Can you work these out from the model? Positions are in its coordinate system, mm. A direction names the side the tool comes from. Round coordinates to 2 decimals unless told otherwise and drop trailing zeros. Order: outer loops, then holes, each group sorted by start corner. A loop starts at its lowest first (then second) coordinate and runs counter-clockwise, first axis right, second up. Notation, with made-up numbers: M -29.5,43 L -0.5,43 A17 cw -0.5,74 Z; hole C 71.5,-31 d4. An arc over 180 degrees is marked long. One line per question, with ' | ' between items.
```python
from build123d import *

# Parameters (mm, degrees)
SKETCH1_W           = 20
SKETCH1_H           = 20
BOSS_EXTRUDE1_DEPTH = 1
CUT_EXTRUDE1_DEPTH  = 1
FILL_START          = -1
FILL_PATTERN1_DEPTH = 2
SKETCH2_W           = 20
SKETCH2_H           = 20
BOSS_EXTRUDE2_DEPTH = 1


# Read off the part's stored shape, not the designer's step: Fill Pattern1
with BuildPart() as part:
    # Sketch1 → Boss-Extrude1 (new, symmetric)
    with BuildSketch(Plane(origin=(0, 0, 0), x_dir=(1, 0, 0), z_dir=(0, 1, 0))):
        Rectangle(SKETCH1_W, SKETCH1_H)
    extrude(amount=BOSS_EXTRUDE1_DEPTH, both=True)

    # Sketch1<4> → Cut-Extrude1 (cut, symmetric)
    with BuildSketch(Plane(origin=(0, 0, 0), x_dir=(1, 0, 0), z_dir=(0, 1, 0))):
        with BuildLine():
            Line((0.5, 2.5), (0.5, -2.5))
            ThreePointArc((0.5, -2.5), (0, -3), (-0.5, -2.5))
            Line((-0.5, -2.5), (-0.5, 2.5))
            ThreePointArc((-0.5, 2.5), (0, 3), (0.5, 2.5))
        make_face()
    extrude(amount=CUT_EXTRUDE1_DEPTH, both=True, mode=Mode.SUBTRACT)

    # Fill Pattern1 outline → Fill Pattern1 (cut)
    with BuildSketch(Plane(origin=(0, 0, 0), x_dir=(1, 0, 0), z_dir=(0, 1, 0)).offset(FILL_START)):
        with BuildLine():
            Line((0.5, -10), (0.5, -6.160254038))
            ThreePointArc((0.5, -6.160254038), (0, -5.660254038), (-0.5, -6.160254038))
            Line((-0.5, -6.160254038), (-0.5, -10))
            Line((-0.5, -10), (0.5, -10))
        make_face()
        with BuildLine():
            ThreePointArc((2.597603377, -10), (2.5, -9.990381057), (2.402396623, -10))
            Line((2.402396623, -10), (2.597603377, -10))
        make_face()
        with BuildLine():
            Line((-2.597603377, -10), (-2.402396623, -10))
            ThreePointArc((-2.402396623, -10), (-2.5, -9.990381057), (-2.597603377, -10))
        make_face()
        with BuildLine():
            Line((4.5, -6.160254038), (4.5, -10))
            Line((4.5, -10), (5.5, -10))
            Line((5.5, -10), (5.5, -6.160254038))
            ThreePointArc((5.5, -6.160254038), (5, -5.660254038), (4.5, -6.160254038))
        make_face()
        with BuildLine():
            Line((-5.5, -10), (-4.5, -10))
            Line((-4.5, -10), (-4.5, -6.160254038))
            ThreePointArc((-4.5, -6.160254038), (-5, -5.660254038), (-5.5, -6.160254038))
            Line((-5.5, -6.160254038), (-5.5, -10))
        make_face()
        with BuildLine():
            ThreePointArc((7.597603377, -10), (7.5, -9.990381057), (7.402396623, -10))
            Line((7.402396623, -10), (7.597603377, -10))
        make_face()
        with BuildLine():
            Line((-7.597603377, -10), (-7.402396623, -10))
            ThreePointArc((-7.402396623, -10), (-7.5, -9.990381057), (-7.597603377, -10))
        make_face()
        with BuildLine():
            Line((9.5, -6.160254038), (9.5, -10))
            Line((9.5, -10), (10, -10))
            Line((10, -10), (10, -5.660254038))
            ThreePointArc((10, -5.660254038), (9.646446609, -5.806700647), (9.5, -6.160254038))
        make_face()
        with BuildLine():
            Line((-10, -10), (-9.5, -10))
            Line((-9.5, -10), (-9.5, -6.160254038))
            ThreePointArc((-9.5, -6.160254038), (-9.646446609, -5.806700647), (-10, -5.660254038))
            Line((-10, -5.660254038), (-10, -10))
        make_face()
        with BuildLine():
            ThreePointArc((9.5, -2.5), (9.646446609, -2.853553391), (10, -3))
            Line((10, -3), (10, 3))
            ThreePointArc((10, 3), (9.646446609, 2.853553391), (9.5, 2.5))
            Line((9.5, 2.5), (9.5, -2.5))
        make_face()
        with BuildLine():
            Line((-10, 3), (-10, -3))
            ThreePointArc((-10, -3), (-9.646446609, -2.853553391), (-9.5, -2.5))
            Line((-9.5, -2.5), (-9.5, 2.5))
            ThreePointArc((-9.5, 2.5), (-9.646446609, 2.853553391), (-10, 3))
        make_face()
        with BuildLine():
            ThreePointArc((9.5, 6.160254038), (9.646446609, 5.806700647), (10, 5.660254038))
            Line((10, 5.660254038), (10, 10))
            Line((10, 10), (9.5, 10))
            Line((9.5, 10), (9.5, 6.160254038))
        make_face()
        with BuildLine():
            Line((-10, 10), (-10, 5.660254038))
            ThreePointArc((-10, 5.660254038), (-9.646446609, 5.806700647), (-9.5, 6.160254038))
            Line((-9.5, 6.160254038), (-9.5, 10))
            Line((-9.5, 10), (-10, 10))
        make_face()
        with BuildLine():
            ThreePointArc((7.402396623, 10), (7.5, 9.990381057), (7.597603377, 10))
            Line((7.597603377, 10), (7.402396623, 10))
        make_face()
        with BuildLine():
            Line((-7.402396623, 10), (-7.597603377, 10))
            ThreePointArc((-7.597603377, 10), (-7.5, 9.990381057), (-7.402396623, 10))
        make_face()
        with BuildLine():
            Line((5.5, 6.160254038), (5.5, 10))
            Line((5.5, 10), (4.5, 10))
            Line((4.5, 10), (4.5, 6.160254038))
            ThreePointArc((4.5, 6.160254038), (5, 5.660254038), (5.5, 6.160254038))
        make_face()
        with BuildLine():
            Line((-4.5, 10), (-5.5, 10))
            Line((-5.5, 10), (-5.5, 6.160254038))
            ThreePointArc((-5.5, 6.160254038), (-5, 5.660254038), (-4.5, 6.160254038))
            Line((-4.5, 6.160254038), (-4.5, 10))
        make_face()
        with BuildLine():
            ThreePointArc((2.402396623, 10), (2.5, 9.990381057), (2.597603377, 10))
            Line((2.597603377, 10), (2.402396623, 10))
        make_face()
        with BuildLine():
            Line((-2.402396623, 10), (-2.597603377, 10))
            ThreePointArc((-2.597603377, 10), (-2.5, 9.990381057), (-2.402396623, 10))
        make_face()
        with BuildLine():
            Line((0.5, 6.160254038), (0.5, 10))
            Line((0.5, 10), (-0.5, 10))
            Line((-0.5, 10), (-0.5, 6.160254038))
            ThreePointArc((-0.5, 6.160254038), (0, 5.660254038), (0.5, 6.160254038))
        make_face()
        with BuildLine():
            Line((8, -6.830127019), (8, -1.830127019))
            ThreePointArc((8, -1.830127019), (7.5, -1.330127019), (7, -1.830127019))
            Line((7, -1.830127019), (7, -6.830127019))
            ThreePointArc((7, -6.830127019), (7.5, -7.330127019), (8, -6.830127019))
        make_face()
        with BuildLine():
            Line((8, 1.830127019), (8, 6.830127019))
            ThreePointArc((8, 6.830127019), (7.5, 7.330127019), (7, 6.830127019))
            Line((7, 6.830127019), (7, 1.830127019))
            ThreePointArc((7, 1.830127019), (7.5, 1.330127019), (8, 1.830127019))
        make_face()
        with BuildLine():
            Line((5.5, -2.5), (5.5, 2.5))
            ThreePointArc((5.5, 2.5), (5, 3), (4.5, 2.5))
            Line((4.5, 2.5), (4.5, -2.5))
            ThreePointArc((4.5, -2.5), (5, -3), (5.5, -2.5))
        make_face()
        with BuildLine():
            Line((-7, 1.830127019), (-7, 6.830127019))
            ThreePointArc((-7, 6.830127019), (-7.5, 7.330127019), (-8, 6.830127019))
            Line((-8, 6.830127019), (-8, 1.830127019))
            ThreePointArc((-8, 1.830127019), (-7.5, 1.330127019), (-7, 1.830127019))
        make_face()
        with BuildLine():
            Line((-7, -6.830127019), (-7, -1.830127019))
            ThreePointArc((-7, -1.830127019), (-7.5, -1.330127019), (-8, -1.830127019))
            Line((-8, -1.830127019), (-8, -6.830127019))
            ThreePointArc((-8, -6.830127019), (-7.5, -7.330127019), (-7, -6.830127019))
        make_face()
        with BuildLine():
            Line((-4.5, -2.5), (-4.5, 2.5))
            ThreePointArc((-4.5, 2.5), (-5, 3), (-5.5, 2.5))
            Line((-5.5, 2.5), (-5.5, -2.5))
            ThreePointArc((-5.5, -2.5), (-5, -3), (-4.5, -2.5))
        make_face()
        with BuildLine():
            Line((3, 1.830127019), (3, 6.830127019))
            ThreePointArc((3, 6.830127019), (2.5, 7.330127019), (2, 6.830127019))
            Line((2, 6.830127019), (2, 1.830127019))
            ThreePointArc((2, 1.830127019), (2.5, 1.330127019), (3, 1.830127019))
        make_face()
        with BuildLine():
            Line((3, -6.830127019), (3, -1.830127019))
            ThreePointArc((3, -1.830127019), (2.5, -1.330127019), (2, -1.830127019))
            Line((2, -1.830127019), (2, -6.830127019))
            ThreePointArc((2, -6.830127019), (2.5, -7.330127019), (3, -6.830127019))
        make_face()
        with BuildLine():
            Line((-2, 1.830127019), (-2, 6.830127019))
            ThreePointArc((-2, 6.830127019), (-2.5, 7.330127019), (-3, 6.830127019))
            Line((-3, 6.830127019), (-3, 1.830127019))
            ThreePointArc((-3, 1.830127019), (-2.5, 1.330127019), (-2, 1.830127019))
        make_face()
        with BuildLine():
            Line((-2, -6.830127019), (-2, -1.830127019))
            ThreePointArc((-2, -1.830127019), (-2.5, -1.330127019), (-3, -1.830127019))
            Line((-3, -1.830127019), (-3, -6.830127019))
            ThreePointArc((-3, -6.830127019), (-2.5, -7.330127019), (-2, -6.830127019))
        make_face()
    extrude(amount=FILL_PATTERN1_DEPTH, mode=Mode.SUBTRACT)

    # Sketch2 → Boss-Extrude2 (add, symmetric)
    with BuildSketch(Plane(origin=(0, 0, 0), x_dir=(1, 0, 0), z_dir=(0, 1, 0))):
        with Locations((-20, 0)):
            Rectangle(SKETCH2_W, SKETCH2_H)
        with Locations((20, 0)):
            Rectangle(SKETCH2_W, SKETCH2_H)
    extrude(amount=BOSS_EXTRUDE2_DEPTH, both=True)


solid = part.part
```
(1) Will this pin go through, and if not, where does the flat tip stop? pin 1 Ø2 at (x, z) = (0, -0.5) entering from +Y.
Final values:
pin 1: y = 1
(2) If we section it at A-A on z = 4.5: Please give me the cut outline in (x, y), plus the area to 3 significant figures.
Final values:
outline: M -30,-1 L -8,-1 L -8,1 L -30,1 Z; M -7,-1 L -3,-1 L -3,1 L -7,1 Z; M -2,-1 L 2,-1 L 2,1 L -2,1 Z; M 3,-1 L 7,-1 L 7,1 L 3,1 Z; M 8,-1 L 30,-1 L 30,1 L 8,1 Z | area: 112 mm^2
(3) Thinking about a two-plate mould opening in Z: for faces 5 (the cylindrical face through (0.01, -0.01, 5.66)), 6 (the cylindrical face through (-7.49, -0.01, 1.33)), 7 (the flat face through (-30, 0, 0)), which applies, released by +Z, released by -Z, zero draft, split by the parting line, or undercut?
Final values:
face 5: released by +Z | face 6: undercut | face 7: zero draft
(4) If we section it at B-B on z = -8: Please give me the cut outline in (x, y).
Final values:
outline: M -30,-1 L -10,-1 L -10,1 L -30,1 Z; M -9.5,-1 L -5.5,-1 L -5.5,1 L -9.5,1 Z; M -4.5,-1 L -0.5,-1 L -0.5,1 L -4.5,1 Z; M 0.5,-1 L 4.5,-1 L 4.5,1 L 0.5,1 Z; M 5.5,-1 L 9.5,-1 L 9.5,1 L 5.5,1 Z; M 10,-1 L 30,-1 L 30,1 L 10,1 Z
(5) If we section it at C-C on y = -0.1: State how many separate pieces and enclosed holes the cut face has, plus the area to 3 significant figures.
Final values:
separate pieces: 1 | enclosed holes: 13 | area: 1,100 mm^2
(6) On a 3-axis mill with a long thin cutter (end or side, diameter ignored), from which of +Z, -Z, +X, -X, +Y, -Y can I reach the whole of each face in a straight line? I mean faces 1 (the flat face through (-10, 0, 8)), 2 (the flat face through (-10, 0, -8)), 3 (the cylindrical face through (2.51, -0.01, 1.33)), 4 (the flat face through (0, 1, -5)). Say none if no direction works.
Final values:
face 1: +Z, +Y, -Y | face 2: -Z, +Y, -Y | face 3: +Y, -Y | face 4: +Z, -Z, +X, -X, +Y
(7) Please list where these lines run through material, in increasing order: probe 1 along X at (y, z) = (0.7, 8); probe 2 along X at (y, z) = (0.5, -3.5). Write a range as [from, to].
Final values:
probe 1: [-30, -10], [-9.5, -5.5], [-4.5, -0.5], [0.5, 4.5], [5.5, 9.5], [10, 30] | probe 2: [-30, -8], [-7, -3], [-2, 2], [3, 7], [8, 30]
